```python
from build123d import *

# Parameters (mm, degrees)
SKETCH1_R           = 6.35
SKETCH1_R_2         = 3.5
BOSS_EXTRUDE1_DEPTH = 3.175


with BuildPart() as part:
    # Sketch1 → Boss-Extrude1 (new body)
    with BuildSketch(Plane.XY):
        with BuildLine():
            Line((-31.75, -25.4), (31.75, -25.4))
            Line((31.75, -25.4), (31.75, 177.8))
            ThreePointArc((31.75, 177.8), (13.263638058, 197.742640242), (-8.020889983, 180.818593926))
            Line((-8.020889983, 180.818593926), (-31.75, 25.4))
            Line((-31.75, 25.4), (-31.75, -25.4))
        make_face()
        with Locations((11.75, 177.8)):
            Circle(SKETCH1_R, mode=Mode.SUBTRACT)
        with Locations((-19.05, 12.7)):
            Circle(SKETCH1_R_2, mode=Mode.SUBTRACT)
        with Locations((12.7, 12.7)):
            Circle(SKETCH1_R_2, mode=Mode.SUBTRACT)
        with Locations((12.7, -12.7)):
            Circle(SKETCH1_R_2, mode=Mode.SUBTRACT)
        with Locations((-19.05, -12.7)):
            Circle(SKETCH1_R_2, mode=Mode.SUBTRACT)
        with Locations((11.75, 114.3)):
            Circle(SKETCH1_R_2, mode=Mode.SUBTRACT)
    extrude(amount=BOSS_EXTRUDE1_DEPTH)


solid = part.part
```
Can you work these out from the model? Positions are in its coordinate system, mm. Coordinates: 2 decimals unless noted, no trailing zeros. Loops run counter-clockwise (first coordinate to the right, second up) from the corner with the lowest first, then second, coordinate; pieces in that order, holes last. Notation, with made-up numbers: (16, 39) -> (44, 39) arc R16 cw to (44, 62) -> close; hole circle Ø6 at (12.5, 50.25). An arc over 180 degrees is marked (long way). Put each result on its own line as item: value. Start each with the question number.
Q1. Thinking about a two-plate mould opening in X: for faces 1 (the face through (-17.17, 15.65, 1.57)), 2 (the face through (7, 88, 0)), 3 (the face through (13.681, 197.707, 1.565)), which applies, pulls with the +X half, pulls with the -X half, needs draft (parallel to the pull), parting line crosses it, or undercut?
Q2. I want a section at D-D (y = 114.3). Write out the boundary of the cut face in (x, z) (3 decimals).
Q3. I'm going to push flat-ended pins straight in: P1, Ø5.5, axis at x = 11.75, y = 114.3, coming from the +Z side; P2, Ø8, axis at x = 12.7, y = 12.7, coming from the +Z side (3 decimals). Where does each tip first touch, or does it pass through?
Q4. I want a section at C-C (x = -19.05). Write out the boundary of the cut face in (y, z) (3 decimals), plus the area to 3 significant figures.
Q5. If I drill on line 1 (Y direction, x = 10.5, z = 1.85); line 2 (Y direction, x = 12.7, z = 2.3); line 3 (X direction, y = 115.5, z = 1.95), over which ranges is the centre line in solid material (lowest first)? Write a range as [from, to].
Q6. I want a section at A-A (z = 0.85). Write out the boundary of the cut face in (x, y).
Q7. I want a section at B-B (y = 12.7). Write out the boundary of the cut face in (x, z) (3 decimals), plus the area to 3 significant figures.
Taken from the geometry:
1. face 1: undercut
1. face 2: needs draft
1. face 3: parting line crosses it
2. outline: (-18.177, 0) -> (8.25, 0) -> (8.25, 3.175) -> (-18.177, 3.175) -> close; (15.25, 0) -> (31.75, 0) -> (31.75, 3.175) -> (15.25, 3.175) -> close
3. P1: passes through
3. P2: stops at z = 3.175
4. outline: (-25.4, 0) -> (-16.2, 0) -> (-16.2, 3.175) -> (-25.4, 3.175) -> close; (-9.2, 0) -> (9.2, 0) -> (9.2, 3.175) -> (-9.2, 3.175) -> close; (16.2, 0) -> (108.581, 0) -> (108.581, 3.175) -> (16.2, 3.175) -> close
4. area: 381 mm2
5. line 1: y = [-25.4, -15.42], [-9.98, 9.98], [15.42, 111.03], [117.57, 171.57], [184.03, 197.76]
5. line 2: y = [-25.4, -16.2], [-9.2, 9.2], [16.2, 110.93], [117.67, 171.52], [184.08, 197.78]
5. line 3: x = [-17.99, 8.46], [15.04, 31.75]
6. outline: (-31.75, -25.4) -> (31.75, -25.4) -> (31.75, 177.8) arc R20 ccw to (-8.02, 180.82) -> (-31.75, 25.4) -> close; hole circle Ø7 at (-19.05, -12.7); hole circle Ø7 at (-19.05, 12.7); hole circle Ø12.7 at (11.75, 177.8); hole circle Ø7 at (11.75, 114.3); hole circle Ø7 at (12.7, -12.7); hole circle Ø7 at (12.7, 12.7)
7. outline: (-31.75, 0) -> (-22.55, 0) -> (-22.55, 3.175) -> (-31.75, 3.175) -> close; (-15.55, 0) -> (9.2, 0) -> (9.2, 3.175) -> (-15.55, 3.175) -> close; (16.2, 0) -> (31.75, 0) -> (31.75, 3.175) -> (16.2, 3.175) -> close
7. area: 157 mm2
